Can you work these out from the drawing? Everything is in mm from the part's minimum corner. Round coordinates to 2 decimals unless told otherwise and drop trailing zeros. Loops run counter-clockwise (first coordinate to the right, second up) from the corner with the lowest first, then second, coordinate; pieces in that order, holes last. Notation, with made-up numbers: M -33.5,89 L -12.5,89 A20 ccw -12.5,126 Z; hole C -39,66 d2. An arc over 180 degrees is marked long. Use a Markdown table: item, result.
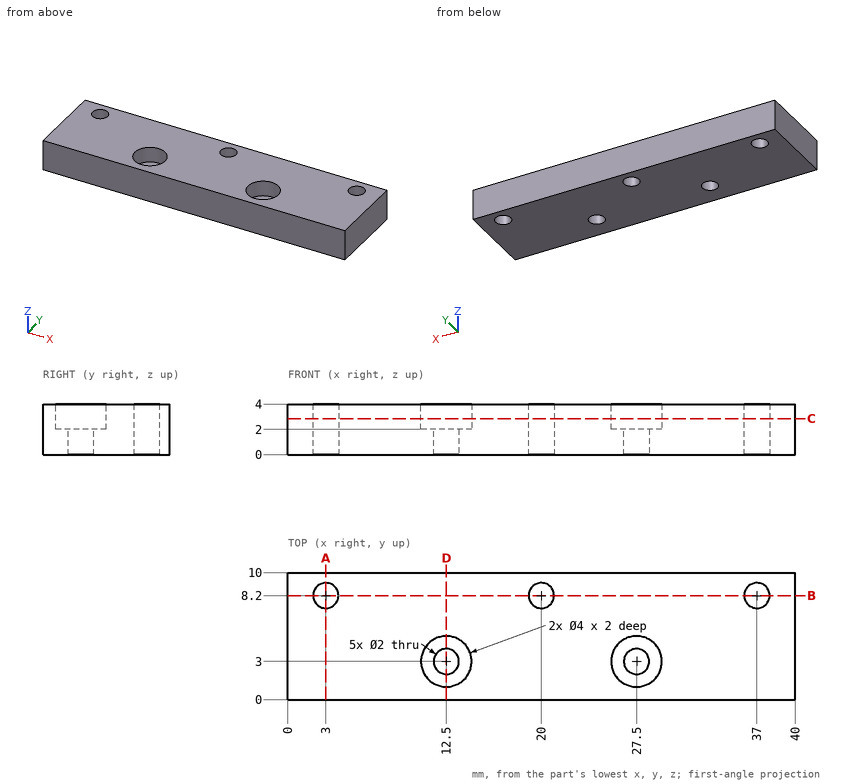
1. Imagine slicing it at B-B, the plane y = 8.2. Write out the boundary of the cut face in (x, z).
Answer sheet:
| item | result |
|---|---|
| outline | M 0,0 L 2,0 L 2,4 L 0,4 Z; M 4,0 L 19,0 L 19,4 L 4,4 Z; M 21,0 L 36,0 L 36,4 L 21,4 Z; M 38,0 L 40,0 L 40,4 L 38,4 Z |
2. For pin 1 Ø4.5 at (x, y) = (27.5, 2.5) entering from +Z; pin 2 Ø1.6 at (x, y) = (37, 8.2) entering from +Z; pin 3 Ø2.5 at (x, y) = (27.5, 3) entering from +Z, each with a flat end and sliding along its axis, tell me the tip position at first contact or that it passes through.
Answer sheet:
| item | result |
|---|---|
| pin 1 | z = 4 |
| pin 2 | through |
| pin 3 | z = 2 |
3. Imagine slicing it at C-C, the plane z = 2.85. Write out the boundary of the cut face in (x, y).
Answer sheet:
| item | result |
|---|---|
| outline | M 0,0 L 40,0 L 40,10 L 0,10 Z; hole C 3,8.2 d2; hole C 12.5,3 d4; hole C 20,8.2 d2; hole C 27.5,3 d4; hole C 37,8.2 d2 |
4. Imagine slicing it at D-D, the plane x = 12.5. Write out the boundary of the cut face in (y, z), then the cut area to 3 significant figures.
Answer sheet:
| item | result |
|---|---|
| outline | M 0,0 L 2,0 L 2,2 L 1,2 L 1,4 L 0,4 Z; M 4,0 L 10,0 L 10,4 L 5,4 L 5,2 L 4,2 Z |
| area | 28.0 mm2 |
5. I need wall thicknesses on probe 1 along X at (y, z) = (8.25, 3.3); probe 2 along Y at (x, z) = (12.5, 2.55); probe 3 along Y at (x, z) = (37, 3.6). Which ranges of each line are inside material? Lowest first, please. Write a range as from..to.
Answer sheet:
| item | result |
|---|---|
| probe 1 | 0..2, 4..19, 21..36, 38..40 |
| probe 2 | 0..1, 5..10 |
| probe 3 | 0..7.2, 9.2..10 |
6. Imagine slicing it at A-A, the plane x = 3. Write out the boundary of the cut face in (y, z), then the cut area to 3 significant figures.
Answer sheet:
| item | result |
|---|---|
| outline | M 0,0 L 7.2,0 L 7.2,4 L 0,4 Z; M 9.2,0 L 10,0 L 10,4 L 9.2,4 Z |
| area | 32.0 mm2 |
